from build123d import *

# Parameters (mm, degrees)
SKETCH1_W           = 55
SKETCH1_H           = 45
BOSS_EXTRUDE1_DEPTH = 5
SKETCH3_W           = 55
SKETCH3_H           = 13
BOSS_EXTRUDE5_DEPTH = 20
CHAMFER1_SIZE       = 8
SKETCH5_R           = 4.5
CUT_EXTRUDE2_DEPTH  = 8
BOSS_EXTRUDE7_DEPTH = 48
CUT_EXTRUDE3_DEPTH  = 71.205777697
CHAMFER2_SIZE       = 3.5
CHAMFER3_SIZE       = 3.5
CHAMFER4_SIZE       = 7
BOSS_EXTRUDE8_DEPTH = 3


with BuildPart() as part:
    # Sketch1 → Boss-Extrude1 (new body)
    with BuildSketch(Plane.XY):
        with Locations((17.145774036, 16.279520652)):
            Rectangle(SKETCH1_W, SKETCH1_H)
    extrude(amount=BOSS_EXTRUDE1_DEPTH)

    # Sketch3 → Boss-Extrude5 (add)
    with BuildSketch(Plane(origin=(0, 0, 0), x_dir=(-1, 0, 0), z_dir=(0, 0, -1))):
        with Locations((-17.145774036, 0.279520652)):
            Rectangle(SKETCH3_W, SKETCH3_H)
    extrude(amount=BOSS_EXTRUDE5_DEPTH)

    # Chamfer1
    chamfer1_edges = [part.edges().sort_by_distance(p)[0] for p in [
        (17.145774036, -6.220479348, 5),
    ]]
    chamfer(chamfer1_edges, length=CHAMFER1_SIZE)

    # Sketch5 → Cut-Extrude2 (cut)
    with BuildSketch(Plane.XZ.offset(6.220479348)):
        with Locations(Location((-0.354225964, -11, 0), (0, 0, 270))):
            Circle(SKETCH5_R)
        with Locations(Location((34.645774036, -11, 0), (0, 0, 270))):
            Circle(SKETCH5_R)
    extrude(amount=-CUT_EXTRUDE2_DEPTH, mode=Mode.SUBTRACT)

    # Sketch7 → Boss-Extrude7 (add)
    with BuildSketch(Plane.ZY.offset(6.854225964)):
        with BuildLine():
            Line((-8.308177677, 10.21387745), (-12.629175087, 12.000050953))
            ThreePointArc((-12.629175087, 12.000050953), (-15.003318067, 13.416764905), (-16.86901604, 15.457060078))
            Line((-16.86901604, 15.457060078), (-15.17096521, 16.605591044))
            ThreePointArc((-15.17096521, 16.605591044), (-1.55, 20.779520652), (-15.17096521, 24.95345026))
            Line((-15.17096521, 24.95345026), (-16.86901604, 26.101981226))
            ThreePointArc((-16.86901604, 26.101981226), (-15.003318067, 28.142276398), (-12.629175087, 29.55899035))
            Line((-12.629175087, 29.55899035), (0, 34.779520652))
            Line((0, 34.779520652), (0, 6.779520652))
            Line((0, 6.779520652), (-8.576470695, 6.779520652))
            ThreePointArc((-8.576470695, 6.779520652), (-7.194534972, 8.39922137), (-8.308177677, 10.21387745))
        make_face()
    extrude(amount=-BOSS_EXTRUDE7_DEPTH)

    # Sketch8 → Cut-Extrude3 (cut, through all)
    with BuildSketch(Plane.ZY.offset(10.354225964)):
        Polygon((0, 34.779520652), (5, 36.846373896), (5, 38.779520652), (0, 38.779520652), align=None)
    extrude(amount=-CUT_EXTRUDE3_DEPTH, mode=Mode.SUBTRACT)

    # Chamfer2
    chamfer2_edges = [part.edges().sort_by_distance(p)[0] for p in [
        (-10.354225964, 6.779520652, -10),
        (-10.354225964, 20.779520652, 0),
    ]]
    chamfer(chamfer2_edges, length=CHAMFER2_SIZE - 0.0001)  # a hair under: the kernel refuses the full size

    # Chamfer3
    chamfer3_edges = [part.edges().sort_by_distance(p)[0] for p in [
        (44.645774036, 20.779520652, 0),
        (44.645774036, 6.779520652, -10),
    ]]
    chamfer(chamfer3_edges, length=CHAMFER3_SIZE - 0.0001)  # a hair under: the kernel refuses the full size

    # Chamfer4
    chamfer4_edges = [part.edges().sort_by_distance(p)[0] for p in [
        (44.645774036, -1.470429348, -20),
        (-10.354225964, -1.470429348, -20),
    ]]
    chamfer(chamfer4_edges, length=CHAMFER4_SIZE)

    # Sketch9 → Boss-Extrude8 (add)
    with BuildSketch(Plane.ZY.offset(6.854225964)):
        with BuildLine():
            Line((-15.17096521, 24.95345026), (-12.313269912, 23.020556683))
            ThreePointArc((-12.313269912, 23.020556683), (-5, 20.779520652), (-12.313269912, 18.538484621))
            Line((-12.313269912, 18.538484621), (-15.17096521, 16.605591044))
            ThreePointArc((-15.17096521, 16.605591044), (-1.55, 20.779520652), (-15.17096521, 24.95345026))
        make_face()
    extrude(amount=-BOSS_EXTRUDE8_DEPTH)


solid = part.part
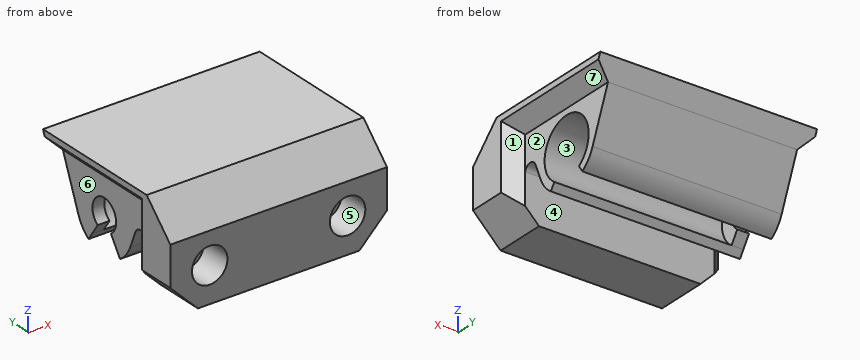
Could you check a few things on this model? Use its own coordinates, in mm. Face numbers are marked on the shaded views. A direction names the side the tool comes from. Give positions to 0.01 mm unless a question says otherwise; leave off trailing zeros. Order: outer loops, then holes, each group sorted by start corner. A loop starts at its lowest first (then second) coordinate and runs counter-clockwise, first axis right, second up.
1. Suppose I cut it at B-B (y = -2). List the corners of the cut face in (x, z) for me, plus the area to 3 significant figures.
2. We'd pull the mould along Y, two halves only. Please class the marked faces 1, 2, 3 and 4: pulls with the +Y half, pulls with the -Y half, needs draft (parallel to the pull), parting line crosses it, or undercut.
3. For the marked faces 5, 6 and 7, which set-ups out of +Z, -Z, +X, -X, +Y, -Y let a thin tool reach every point of the face, with its end or its side?
4. Suppose I cut it at C-C (z = -14). List the corners of the cut face in (x, y) for me.
5. I need wall thicknesses on L1, parallel to X at y = -3.25, z = -11; L2, parallel to Y at x = 35.5, z = -15.25; L3, parallel to Y at x = 6.5, z = -16.75. Which ranges of each line are inside material? Lowest first, please.
6. Suppose I cut it at A-A (x = 26). List the corners of the cut face in (y, z) for me.
7. Will these pins go through, and if not, where does the flat tip stop? P1, Ø8, axis at y = 12, z = -3.5, coming from the +X side; P2, Ø8.5, axis at y = 24, z = -8.5, coming from the +X side; P3, Ø3, axis at x = 0, z = -15, coming from the -Y side; P4, Ø7, axis at y = 20, z = -7, coming from the +X side.
8. Suppose I cut it at D-D (z = 1.25). List the corners of the cut face in (x, y) for me.
Solved:
1. outline: (-10.35, -13) - (-3.35, -20) - (37.65, -20) - (44.65, -13) - (44.65, 1.22) - (-10.35, 1.22) - close; hole circle Ø9 at (-0.35, -11); hole circle Ø9 at (34.65, -11)
1. area: 991 mm2
2. face 1: pulls with the +Y half
2. face 2: needs draft
2. face 3: undercut
2. face 4: undercut
3. face 5: -Y
3. face 6: -Z, -X, +Y
3. face 7: -Z, +X, +Y
4. outline: (-9.35, -6.22) - (-3.71, -6.22) - (-3.71, 1.78) - (3, 1.78) - (3, -6.22) - (31.29, -6.22) - (31.29, 1.78) - (38, 1.78) - (38, -6.22) - (43.65, -6.22) - (43.65, 4.28) - (41.15, 6.78) - (-6.85, 6.78) - (-9.35, 4.28) - close; (-6.85, 12.7) - (41.15, 12.7) - (41.15, 15.26) - (-3.85, 15.26) - (-3.85, 17.4) - (-6.85, 17.4) - close; (-6.85, 24.16) - (-3.85, 24.16) - (-3.85, 26.3) - (41.15, 26.3) - (41.15, 28.86) - (-6.85, 28.86) - close
5. L1: x = -10.35 to -4.85, 4.15 to 30.15, 39.15 to 44.65
5. L2: y = 1.78 to 6.78, 13.62 to 16.55, 25.01 to 27.93
5. L3: y = -6.22 to 6.78, 15.29 to 15.54, 26.02 to 26.27
6. outline: (-6.22, -20) - (6.78, -20) - (6.78, -8.58) arc R1.81 cw to (10.21, -8.31) - (12, -12.63) arc R9.5 ccw to (15.46, -16.87) - (16.61, -15.17) arc R7.45 cw (long way) to (24.95, -15.17) - (26.1, -16.87) arc R9.5 ccw to (29.56, -12.63) - (36.85, 5) - (1.78, 5) - (-6.22, -3) - close
7. P1: stops at x = 41.65
7. P2: stops at x = 41.15
7. P3: stops at y = -6.22
7. P4: stops at x = -3.85
8. outline: (-10.35, -1.97) - (44.65, -1.97) - (44.65, 3.28) - (42.4, 5.53) - (42.4, 35.3) - (-8.1, 35.3) - (-8.1, 5.53) - (-10.35, 3.28) - close
